```python
from build123d import *

# Parameters (mm, degrees)
SKETCH1_W           = 135
SKETCH1_H           = 130
SKETCH1_R           = 2.75
BOSS_EXTRUDE2_DEPTH = 5
FILLET1_R           = 10


with BuildPart() as part:
    # Sketch1 → Boss-Extrude2 (new body)
    with BuildSketch(Plane(origin=(0, 0, 0), x_dir=(1, 0, 0), z_dir=(0, 1, 0))):
        with Locations((67.5, 65)):
            Rectangle(SKETCH1_W, SKETCH1_H)
        with Locations(Location((15, 10, 0), (0, 0, 270))):
            Circle(SKETCH1_R, mode=Mode.SUBTRACT)
        with Locations(Location((47, 10, 0), (0, 0, 270))):
            Circle(SKETCH1_R, mode=Mode.SUBTRACT)
        with Locations(Location((15, 120, 0), (0, 0, 270))):
            Circle(SKETCH1_R, mode=Mode.SUBTRACT)
        with Locations(Location((47, 120, 0), (0, 0, 270))):
            Circle(SKETCH1_R, mode=Mode.SUBTRACT)
        Polygon((20, 102.925904836), (107.925904836, 20), (20, 20), align=None, mode=Mode.SUBTRACT)
        Polygon((27.074095164, 110), (115, 27.074095164), (115, 110), align=None, mode=Mode.SUBTRACT)
    extrude(amount=BOSS_EXTRUDE2_DEPTH)

    # Fillet1
    fillet1_edges = [part.edges().sort_by_distance(p)[0] for p in [
        (0, 2.5, 0),
        (0, 2.5, -130),
    ]]
    fillet(fillet1_edges, radius=FILLET1_R)


solid = part.part
```
CAD build for the part. Positions are in the model's coordinates, mm. A direction names the side the tool comes from. Round coordinates to 2 decimals unless told otherwise and drop trailing zeros. Order: outer loops, then holes, each group sorted by start corner. A loop starts at its lowest first (then second) coordinate and runs counter-clockwise, first axis right, second up. Notation, with made-up numbers: (-14.5, -35.5) - (32.5, -35.5) arc R18 cw to (32.5, -7.5) - close; hole circle Ø6 at (68, -18.75). An arc over 180 degrees is marked (long way). Answer in a Markdown table with one row per item. Add a question column.
(1) Band-saw the part on D-D on z = -107. List the corners of the cut face in (x, y), and give its area (3 significant figures).
(2) Probe L1, parallel to X at y = 1.7, z = -120; L2, parallel to X at y = 2.95, z = -42; L3, parallel to Z at x = 57.5, y = 0.75. List the from-to ranges inside material, lowest first. Write a range as [from, to].
(3) Band-saw the part on A-A on y = 3.3. List the corners of the cut face in (x, z), and give its area (3 significant figures).
(4) Mould opens along X. For faces 1 (the face through (49.727, 2.465, -120.358)), 2 (the face through (67, 0, -66)), 3 (the face through (2.85, 2.54, -126.99)) say: +X half, -X half, draft (parallel to the pull), parting line (faces both ways), or undercut.
(5) Band-saw the part on C-C on x = 97. List the corners of the cut face in (y, z).
(6) Band-saw the part on B-B on z = -46. List the corners of the cut face in (x, y).
(7) 3-axis set-ups, long thin cutter, end or side, ignore diameter. For faces 4 (the face through (70.42, 2.46, -69.12)), 5 (the face through (0, 2, -64)): which of +Z, -Z, +X, -X, +Y, -Y reach the whole face in a straight line?
Data:
| question | item | result |
|---|---|---|
| 1 | outline | (0, 0) - (30.25, 0) - (30.25, 5) - (0, 5) - close; (115, 0) - (135, 0) - (135, 5) - (115, 5) - close |
| 1 | area | 251 mm^2 |
| 2 | L1 | x = [0, 12.25], [17.75, 44.25], [49.75, 135] |
| 2 | L2 | x = [0, 20], [84.6, 99.17], [115, 135] |
| 2 | L3 | z = [-130, -110], [-81.3, -67.56], [-20, 0] |
| 3 | outline | (0, -120) arc R10 ccw to (10, -130) - (135, -130) - (135, 0) - (10, 0) arc R10 ccw to (0, -10) - close; hole circle Ø5.5 at (15, -120); hole circle Ø5.5 at (15, -10); hole (20, -102.93) - (107.93, -20) - (20, -20) - close; hole (27.07, -110) - (115, -110) - (115, -27.07) - close; hole circle Ø5.5 at (47, -120); hole circle Ø5.5 at (47, -10) |
| 3 | area | 10,100 mm^2 |
| 4 | face 1 | undercut |
| 4 | face 2 | draft |
| 4 | face 3 | -X half |
| 5 | outline | (0, -130) - (5, -130) - (5, -110) - (0, -110) - close; (0, -44.05) - (5, -44.05) - (5, -30.3) - (0, -30.3) - close; (0, -20) - (5, -20) - (5, 0) - (0, 0) - close |
| 6 | outline | (0, 0) - (20, 0) - (20, 5) - (0, 5) - close; (80.36, 0) - (94.93, 0) - (94.93, 5) - (80.36, 5) - close; (115, 0) - (135, 0) - (135, 5) - (115, 5) - close |
| 7 | face 4 | +Y, -Y |
| 7 | face 5 | +Z, -Z, -X, +Y, -Y |
